Autodesk Inventor part; units mm, degrees
ref_plane "YZ Plane" through (0, 0, 0) normal (1, 0, 0) x (0, 1, 0)
ref_plane "XZ Plane" through (0, 0, 0) normal (0, 1, 0) x (-1, 0, 0)
ref_plane "XY Plane" through (0, 0, 0) normal (0, 0, 1) x (1, 0, 0)
sketch "スケッチ1" plane through (0, 0, 0) normal (0, 0, 1) x (1, 0, 0)
  circle A0 centre (0, 0) radius 1.5
  dimension "d0" = 3
extrude "押し出し1" add sketch "スケッチ1" along normal blind 6
sketch "スケッチ2" plane through (0, 0, 6) normal (0, 0, 1) x (1, 0, 0)
  circle A0 centre (0, 0) radius 1.5
  circle A1 centre (0, 0) radius 3
  dimension "d3" = 6
extrude "押し出し2" add sketch "スケッチ2" along normal blind 1.75 contours A0 | A1
thread "ねじ1"
chamfer "面取り1" distance 1.5 angle 45 1 edges at (-3, 0, 6)
sketch "スケッチ4" plane through (0, 0, 0) normal (0, 0, -1) x (-1, 0, 0)
  circle A0 centre (0, 0) radius 1.5
extrude "押し出し4" add sketch "スケッチ4" along normal blind 4
sketch "スケッチ5" plane through (0, 0, -4) normal (0, 0, -1) x (-1, 0, 0)
  circle A0 centre (0, 0) radius 1.5
extrude "押し出し5" cut sketch "スケッチ5" against normal blind 2
sketch "スケッチ6" plane through (0, 0, -2) normal (0, 0, -1) x (-1, 0, 0)
  circle A0 centre (0, 0) radius 1.5
extrude "押し出し6" add sketch "スケッチ6" along normal blind 8.25
properties part number "SB　18mm皿ネジ" material "Steel, Mild"
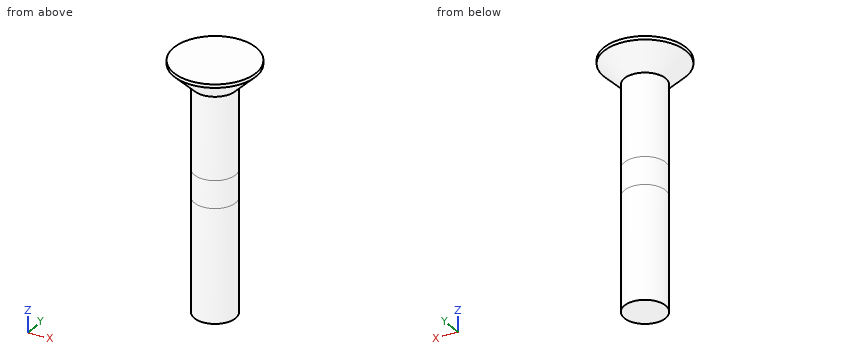
The model under review builds one solid part; all positions refer to its coordinate system, in mm. Round coordinates to 2 decimals unless told otherwise and drop trailing zeros. Order: outer loops, then holes, each group sorted by start corner. A loop starts at its lowest first (then second) coordinate and runs counter-clockwise, first axis right, second up.
(1) Take a section at D-D, the plane z = 6.25. State the section outline as (x, y) points.
Working result:
outline: circle Ø3.5 at (0, 0)
(2) Wall thickness on L1, parallel to Y at x = -0.65, z = -2.75; L2, parallel to Z at x = 0.7, y = 1.4; L3, parallel to Z at x = 1.4, y = 1: over which ranges is each line inside the solid? List them lowest first.
Working result:
L1: y = -1.35 to 1.35
L2: z = 6.06 to 7.75
L3: z = 6.22 to 7.75
(3) For P1, Ø2, axis at x = -1, z = -3.5, coming from the +Y side; P2, Ø2, axis at x = 1.5, y = -1, coming from the -Z side; P3, Ø3, axis at y = -0.5, z = -1, coming from the -X side, all flat-tipped, find the tip position at first contact; note any pin that passes through.
Working result:
P1: stops at y = 1.5
P2: stops at z = -10.25
P3: stops at x = -1.5
(4) Take a section at C-C, the plane z = 0.25. State the section outline as (x, y) points.
Working result:
outline: circle Ø3 at (0, 0)
